from build123d import *

# Parameters (mm, degrees)
F0_R         = 16.51
F1_DEPTH     = 6.35
F2_DEPTH     = 44.45
F3_T1_DEPTH  = 34.29
F3_T3_DEPTH  = 33.02
F3_T5_DEPTH  = 33.02
F3_S9_W      = 5.08
F3_S9_H      = 5.08
F3_T10_DEPTH = 5.08
F3_S15_W     = 5.08
F3_S15_H     = 5.08
F3_T16_DEPTH = 5.08
F3_S21_W     = 5.08
F3_S21_H     = 5.08
F3_T22_DEPTH = 5.08
F3_S27_W     = 5.08
F3_S27_H     = 5.08
F3_T28_DEPTH = 5.08
F3_S33_W     = 5.08
F3_S33_H     = 5.08
F3_T34_DEPTH = 5.08
F3_S39_W     = 5.08
F3_S39_H     = 5.08
F3_T40_DEPTH = 5.08
F3_S45_W     = 5.08
F3_S45_H     = 5.08
F3_T46_DEPTH = 5.08
F3_S51_W     = 5.08
F3_S51_H     = 5.08
F3_T52_DEPTH = 5.08
F4_R         = 3.175
F5_DEPTH     = 25.4


# Not quite as in the source:
# - a fillet or chamfer that OpenCascade refuses, or shapes differently, is made with other operations: its cross-section is extruded or revolved along the edge and cut away or added


with BuildPart() as f1:
    # F0 (on Front) → F1 (new body)
    with BuildSketch(Plane.XZ):
        Circle(F0_R)
    extrude(amount=F1_DEPTH)

    # F0 (on Front) → F2 (join)
    with BuildSketch(Plane.XZ):
        Polygon((21.59, 21.59), (0, 21.59), (-21.59, 21.59), (-21.59, 0), (-21.59, -21.59), (21.59, -21.59), align=None)
        Circle(F0_R, mode=Mode.SUBTRACT)
    extrude(amount=F2_DEPTH)

    # F3: fillet of radius 5.08 on 13 edges, made by hand

    # F3_s2 → F3_t1 (cut)
    with BuildSketch(Plane.XZ.offset(5.08)):
        with BuildLine():
            ThreePointArc((16.51, 21.59), (20.1021024484, 20.1021024484), (21.59, 16.51))
            Line((21.59, 16.51), (21.59, 21.59))
            Line((21.59, 21.59), (16.51, 21.59))
        make_face()
        with BuildLine():
            ThreePointArc((-16.51, 21.59), (-20.1021024484, 20.1021024484), (-21.59, 16.51))
            Line((-21.59, 16.51), (-21.59, 21.59))
            Line((-21.59, 21.59), (-16.51, 21.59))
        make_face()
        with BuildLine():
            ThreePointArc((-21.59, -16.51), (-20.1021024484, -20.1021024484), (-16.51, -21.59))
            Line((-16.51, -21.59), (-21.59, -21.59))
            Line((-21.59, -21.59), (-21.59, -16.51))
        make_face()
        with BuildLine():
            ThreePointArc((16.51, -21.59), (20.1021024484, -20.1021024484), (21.59, -16.51))
            Line((21.59, -16.51), (21.59, -21.59))
            Line((21.59, -21.59), (16.51, -21.59))
        make_face()
    extrude(amount=F3_T1_DEPTH, mode=Mode.SUBTRACT)

    # F3_s4 → F3_t3 (cut)
    with BuildSketch(Plane.YZ.offset(-16.51)):
        with BuildLine():
            ThreePointArc((0, -16.51), (-1.4878975516, -20.1021024484), (-5.08, -21.59))
            Line((-5.08, -21.59), (0, -21.59))
            Line((0, -21.59), (0, -16.51))
        make_face()
        with BuildLine():
            ThreePointArc((0, 16.51), (-1.4878975516, 20.1021024484), (-5.08, 21.59))
            Line((-5.08, 21.59), (0, 21.59))
            Line((0, 21.59), (0, 16.51))
        make_face()
        with BuildLine():
            ThreePointArc((-39.37, -21.59), (-42.9621024484, -20.1021024484), (-44.45, -16.51))
            Line((-44.45, -16.51), (-44.45, -21.59))
            Line((-44.45, -21.59), (-39.37, -21.59))
        make_face()
        with BuildLine():
            ThreePointArc((-39.37, 21.59), (-42.9621024484, 20.1021024484), (-44.45, 16.51))
            Line((-44.45, 16.51), (-44.45, 21.59))
            Line((-44.45, 21.59), (-39.37, 21.59))
        make_face()
    extrude(amount=F3_T3_DEPTH, mode=Mode.SUBTRACT)

    # F3_s6 → F3_t5 (cut)
    with BuildSketch(Plane.XY.offset(-16.51)):
        with BuildLine():
            ThreePointArc((16.51, 0), (20.1021024484, -1.4878975516), (21.59, -5.08))
            Line((21.59, -5.08), (21.59, 0))
            Line((21.59, 0), (16.51, 0))
        make_face()
        with BuildLine():
            ThreePointArc((-16.51, 0), (-20.1021024484, -1.4878975516), (-21.59, -5.08))
            Line((-21.59, -5.08), (-21.59, 0))
            Line((-21.59, 0), (-16.51, 0))
        make_face()
        with BuildLine():
            ThreePointArc((21.59, -39.37), (20.1021024484, -42.9621024484), (16.51, -44.45))
            Line((16.51, -44.45), (21.59, -44.45))
            Line((21.59, -44.45), (21.59, -39.37))
        make_face()
        with BuildLine():
            ThreePointArc((-21.59, -39.37), (-20.1021024484, -42.9621024484), (-16.51, -44.45))
            Line((-16.51, -44.45), (-21.59, -44.45))
            Line((-21.59, -44.45), (-21.59, -39.37))
        make_face()
    extrude(amount=F3_T5_DEPTH, mode=Mode.SUBTRACT)


with BuildPart() as f3_tool8:
    # F3_s9 → F3_t10 (new body)
    with BuildSketch(Plane.XZ.offset(5.08)):
        with Locations((19.05, 19.05)):
            Rectangle(F3_S9_W, F3_S9_H)
    extrude(amount=-F3_T10_DEPTH)

    # F3_s11 → F3_t12 (revolve, cut)
    with BuildSketch(Plane(origin=(16.51, -5.08, 16.51), x_dir=(-0.7071067812, 0, -0.7071067812), z_dir=(0.7071067812, 0, -0.7071067812))):
        with BuildLine():
            ThreePointArc((0, -5.08), (5.08, 0), (0, 5.08))
            Line((0, 5.08), (0, -5.08))
        make_face()
    revolve(axis=Axis((16.51, -5.08, 16.51), (0, 1, 0)), mode=Mode.SUBTRACT)


with BuildPart() as f1_1:
    add(f1.part)

    # F3_t7: cut F3_tool8
    add(f3_tool8.part, mode=Mode.SUBTRACT)


with BuildPart() as f3_tool14:
    # F3_s15 → F3_t16 (new body)
    with BuildSketch(Plane.XY.offset(16.51)):
        with Locations((19.05, -41.91)):
            Rectangle(F3_S15_W, F3_S15_H)
    extrude(amount=F3_T16_DEPTH)

    # F3_s17 → F3_t18 (revolve, cut)
    with BuildSketch(Plane(origin=(16.51, -39.37, 16.51), x_dir=(-0.7071067812, 0.7071067812, 0), z_dir=(0.7071067812, 0.7071067812, 0))):
        with BuildLine():
            ThreePointArc((0, -5.08), (5.08, 0), (0, 5.08))
            Line((0, 5.08), (0, -5.08))
        make_face()
    revolve(axis=Axis((16.51, -39.37, 16.51), (0, 0, 1)), mode=Mode.SUBTRACT)


with BuildPart() as f1_2:
    add(f1_1.part)

    # F3_t13: cut F3_tool14
    add(f3_tool14.part, mode=Mode.SUBTRACT)


with BuildPart() as f3_tool20:
    # F3_s21 → F3_t22 (new body)
    with BuildSketch(Plane.XZ.offset(5.08)):
        with Locations((-19.05, 19.05)):
            Rectangle(F3_S21_W, F3_S21_H)
    extrude(amount=-F3_T22_DEPTH)

    # F3_s23 → F3_t24 (revolve, cut)
    with BuildSketch(Plane(origin=(-16.51, -5.08, 16.51), x_dir=(0.7071067812, 0, -0.7071067812), z_dir=(0.7071067812, 0, 0.7071067812))):
        with BuildLine():
            ThreePointArc((0, -5.08), (5.08, 0), (0, 5.08))
            Line((0, 5.08), (0, -5.08))
        make_face()
    revolve(axis=Axis((-16.51, -5.08, 16.51), (0, 1, 0)), mode=Mode.SUBTRACT)


with BuildPart() as f1_3:
    add(f1_2.part)

    # F3_t19: cut F3_tool20
    add(f3_tool20.part, mode=Mode.SUBTRACT)


with BuildPart() as f3_tool26:
    # F3_s27 → F3_t28 (new body)
    with BuildSketch(Plane.XY.offset(16.51)):
        with Locations((-19.05, -41.91)):
            Rectangle(F3_S27_W, F3_S27_H)
    extrude(amount=F3_T28_DEPTH)

    # F3_s29 → F3_t30 (revolve, cut)
    with BuildSketch(Plane(origin=(-16.51, -39.37, 16.51), x_dir=(0.7071067812, 0.7071067812, 0), z_dir=(0.7071067812, -0.7071067812, 0))):
        with BuildLine():
            ThreePointArc((0, -5.08), (5.08, 0), (0, 5.08))
            Line((0, 5.08), (0, -5.08))
        make_face()
    revolve(axis=Axis((-16.51, -39.37, 16.51), (0, 0, 1)), mode=Mode.SUBTRACT)


with BuildPart() as f1_4:
    add(f1_3.part)

    # F3_t25: cut F3_tool26
    add(f3_tool26.part, mode=Mode.SUBTRACT)


with BuildPart() as f3_tool32:
    # F3_s33 → F3_t34 (new body)
    with BuildSketch(Plane.XZ.offset(5.08)):
        with Locations((-19.05, -19.05)):
            Rectangle(F3_S33_W, F3_S33_H)
    extrude(amount=-F3_T34_DEPTH)

    # F3_s35 → F3_t36 (revolve, cut)
    with BuildSketch(Plane(origin=(-16.51, -5.08, -16.51), x_dir=(0.7071067812, 0, 0.7071067812), z_dir=(-0.7071067812, 0, 0.7071067812))):
        with BuildLine():
            ThreePointArc((0, -5.08), (5.08, 0), (0, 5.08))
            Line((0, 5.08), (0, -5.08))
        make_face()
    revolve(axis=Axis((-16.51, -5.08, -16.51), (0, 1, 0)), mode=Mode.SUBTRACT)


with BuildPart() as f1_5:
    add(f1_4.part)

    # F3_t31: cut F3_tool32
    add(f3_tool32.part, mode=Mode.SUBTRACT)


with BuildPart() as f3_tool38:
    # F3_s39 → F3_t40 (new body)
    with BuildSketch(Plane.YZ.offset(-16.51)):
        with Locations((-41.91, -19.05)):
            Rectangle(F3_S39_W, F3_S39_H)
    extrude(amount=-F3_T40_DEPTH)

    # F3_s41 → F3_t42 (revolve, cut)
    with BuildSketch(Plane(origin=(-16.51, -39.37, -16.51), x_dir=(0, 0.7071067812, 0.7071067812), z_dir=(0, -0.7071067812, 0.7071067812))):
        with BuildLine():
            ThreePointArc((0, -5.08), (5.08, 0), (0, 5.08))
            Line((0, 5.08), (0, -5.08))
        make_face()
    revolve(axis=Axis((-16.51, -39.37, -16.51), (-1, 0, 0)), mode=Mode.SUBTRACT)


with BuildPart() as f1_6:
    add(f1_5.part)

    # F3_t37: cut F3_tool38
    add(f3_tool38.part, mode=Mode.SUBTRACT)


with BuildPart() as f3_tool44:
    # F3_s45 → F3_t46 (new body)
    with BuildSketch(Plane.XZ.offset(5.08)):
        with Locations((19.05, -19.05)):
            Rectangle(F3_S45_W, F3_S45_H)
    extrude(amount=-F3_T46_DEPTH)

    # F3_s47 → F3_t48 (revolve, cut)
    with BuildSketch(Plane(origin=(16.51, -5.08, -16.51), x_dir=(-0.7071067812, 0, 0.7071067812), z_dir=(-0.7071067812, 0, -0.7071067812))):
        with BuildLine():
            ThreePointArc((0, -5.08), (5.08, 0), (0, 5.08))
            Line((0, 5.08), (0, -5.08))
        make_face()
    revolve(axis=Axis((16.51, -5.08, -16.51), (0, 1, 0)), mode=Mode.SUBTRACT)


with BuildPart() as f1_7:
    add(f1_6.part)

    # F3_t43: cut F3_tool44
    add(f3_tool44.part, mode=Mode.SUBTRACT)


with BuildPart() as f3_tool50:
    # F3_s51 → F3_t52 (new body)
    with BuildSketch(Plane.XY.offset(-16.51)):
        with Locations((19.05, -41.91)):
            Rectangle(F3_S51_W, F3_S51_H)
    extrude(amount=-F3_T52_DEPTH)

    # F3_s53 → F3_t54 (revolve, cut)
    with BuildSketch(Plane(origin=(16.51, -39.37, -16.51), x_dir=(-0.7071067812, 0.7071067812, 0), z_dir=(-0.7071067812, -0.7071067812, 0))):
        with BuildLine():
            ThreePointArc((0, -5.08), (5.08, 0), (0, 5.08))
            Line((0, 5.08), (0, -5.08))
        make_face()
    revolve(axis=Axis((16.51, -39.37, -16.51), (0, 0, -1)), mode=Mode.SUBTRACT)


with BuildPart() as f1_8:
    add(f1_7.part)

    # F3_t49: cut F3_tool50
    add(f3_tool50.part, mode=Mode.SUBTRACT)

    # F3_s55 → F3_t56 (revolve, cut)
    with BuildSketch(Plane.XY):
        with BuildLine():
            ThreePointArc((21.59, -44.45), (17.9978975516, -42.9621024484), (16.51, -39.37))
            Line((16.51, -39.37), (16.51, -44.45))
            Line((16.51, -44.45), (21.59, -44.45))
        make_face()
    revolve(axis=Axis((0, -44.45, 0), (0, -1, 0)), mode=Mode.SUBTRACT)

    # F4 (on face) → F5 (cut)
    with BuildSketch(Plane(origin=(0, 0, 0), x_dir=(-1, 0, 0), z_dir=(0, 1, 0))):
        with Locations((-8.255, 0)):
            Circle(F4_R)
        with Locations((8.255, 0)):
            Circle(F4_R)
    extrude(amount=-F5_DEPTH, mode=Mode.SUBTRACT)


solid = f1_8.part
Could you check a few things on this model? Use its own coordinates, in mm. A direction names the side the tool comes from. Give positions to 0.01 mm unless a question says otherwise; leave off trailing zeros. Order: outer loops, then holes, each group sorted by start corner. A loop starts at its lowest first (then second) coordinate and runs counter-clockwise, first axis right, second up. Notation, with made-up numbers: (9.25, -27.75) - (49.25, -27.75) arc R28 ccw to (49.25, 10.25) - close; hole circle Ø7 at (29, 66.5). An arc over 180 degrees is marked (long way). One line per question, with ' | ' between items. Start each with the question number.
Item 1: I want a section at A-A on y = -10.5. Write out the boundary of the cut face in (x, z), then the cut area to 3 significant figures.
Item 2: I need wall thicknesses on probe 1 along Z at (x, y) = (-0.5, -13.5); probe 2 along Y at (x, z) = (-6.5, -8.5); probe 3 along X at (y, z) = (-33.5, 4). Which ranges of each line are inside material? Lowest first, please. Write a range as [from, to].
Item 3: I'm going to push flat-ended pins straight in: pin 1 Ø5 at (x, z) = (-8, 10) entering from -Y; pin 2 Ø1.5 at (x, z) = (16.5, -10.5) entering from -Y. Where does each tip first touch, or does it pass through?
Item 4: I want a section at C-C on x = 0. Write out the boundary of the cut face in (y, z), then the cut area to 3 significant figures.
Item 5: I want a section at B-B on z = 0. Write out the boundary of the cut face in (x, y).
Item 6: Thinking about a two-plate mould opening in X: for faces 3 (the flat face through (0, -6.35, 0)), 4 (the cylindrical face through (-20.062, -1.449, -0.231)), 5 (the flat face through (0, -22, 21.59)), which applies, pulls with the +X half, pulls with the -X half, needs draft (parallel to the pull), parting line crosses it, or undercut?
Item 7: For faces 1 (the cylindrical face through (-20.7, -42.24, -0.23)), 2 (the cylindrical face through (15.748, -22.629, 4.959)), which set-ups out of +Z, -Z, +X, -X, +Y, -Y let a thin tool reach every point of the face, with its end or its side?
Verdict:
1) outline: (-21.59, -16.51) arc R5.08 ccw to (-16.51, -21.59) - (16.51, -21.59) arc R5.08 ccw to (21.59, -16.51) - (21.59, 16.51) arc R5.08 ccw to (16.51, 21.59) - (-16.51, 21.59) arc R5.08 ccw to (-21.59, 16.51) - close; hole circle Ø33.02 at (0, 0) | area: 986 mm^2
2) probe 1: [-21.59, -16.5], [16.5, 21.59] | probe 2: [-6.35, 0] | probe 3: [-21.59, -16.02], [16.02, 21.59]
3) pin 1: y = -6.35 | pin 2: y = -44.29
4) outline: (-43.77, -19.05) arc R5.08 ccw to (-39.37, -21.59) - (-5.08, -21.59) arc R5.08 ccw to (0, -16.51) - (0, 16.51) arc R5.08 ccw to (-5.08, 21.59) - (-39.37, 21.59) arc R5.08 ccw to (-43.77, 19.05) arc R5.08 ccw to (-39.37, 16.51) - (-6.35, 16.51) - (-6.35, -16.51) - (-39.37, -16.51) arc R5.08 ccw to start | area: 630 mm^2
5) outline: (-21.59, -39.37) arc R5.08 ccw to (-19.05, -43.77) arc R5.08 ccw to (-16.51, -39.37) - (-16.51, -6.35) - (-11.43, -6.35) - (-11.43, 0) - (-16.51, 0) arc R5.08 ccw to (-21.59, -5.08) - close; (-5.08, -6.35) - (5.08, -6.35) - (5.08, 0) - (-5.08, 0) - close; (11.43, -6.35) - (16.51, -6.35) - (16.51, -39.37) arc R5.08 ccw to (19.05, -43.77) arc R5.08 ccw to (21.59, -39.37) - (21.59, -5.08) arc R5.08 ccw to (16.51, 0) - (11.43, 0) - close
6) face 3: undercut | face 4: pulls with the -X half | face 5: needs draft
7) face 1: +Z, -Z, -X, -Y | face 2: -Y
